Part model, mm, in its own coordinate system. Give positions to 0.01 mm unless a question says otherwise; leave off trailing zeros. Order: outer loops, then holes, each group sorted by start corner. A loop starts at its lowest first (then second) coordinate and runs counter-clockwise, first axis right, second up.
1. Slice it at C-C on z = 3.5. Give the number of separate pieces and of enclosed holes in the cut face, and give its area (3 significant figures).
2. Probe line 1 (Y direction, x = 0, z = 4.5); line 2 (X direction, y = -6.5, z = 3.5). List the from-to ranges inside material, lowest first.
3. Slice it at A-A on y = 44.45. List the corners of the cut face in (x, z), and give its area (3 significant figures).
4. Slice it at D-D on x = 0. List the corners of the cut face in (y, z).
5. Drop a flat-ended pin along its axis: pin 1 Ø5.5 at (x, y) = (-44.45, 0) entering from +Z. Give the stop position or say it passes through.
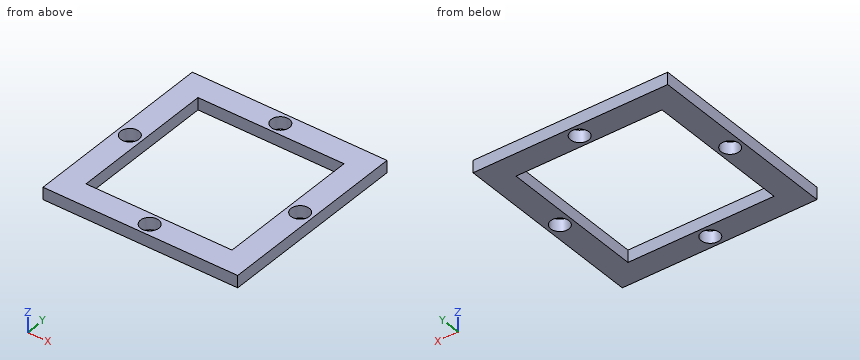
from build123d import *

# Parameters (mm, degrees)
F0_W     = 101.6
F0_H     = 101.6
F0_W_2   = 76.2
F0_H_2   = 76.2
F1_DEPTH = 6.35
F3_D     = 9.525
F3_DEPTH = 12.7


with BuildPart() as f1:
    # F0 (on Top) → F1 (new body)
    with BuildSketch(Plane.XY):
        Rectangle(F0_W, F0_H)
        Rectangle(F0_W_2, F0_H_2, mode=Mode.SUBTRACT)
    extrude(amount=F1_DEPTH)

    # F3
    with Locations(Plane.XY.offset(6.35)):
        with Locations((0, 44.45), (-44.45, 0), (44.45, 0), (0, -44.45)):
            Hole(F3_D / 2, depth=F3_DEPTH)


solid = f1.part
Data:
1. separate pieces: 1
1. enclosed holes: 5
1. area: 4,230 mm2
2. line 1: y = -50.8 to -49.21, -39.69 to -38.1, 38.1 to 39.69, 49.21 to 50.8
2. line 2: x = -50.8 to -38.1, 38.1 to 50.8
3. outline: (-50.8, 0) - (-4.76, 0) - (-4.76, 6.35) - (-50.8, 6.35) - close; (4.76, 0) - (50.8, 0) - (50.8, 6.35) - (4.76, 6.35) - close
3. area: 585 mm2
4. outline: (-50.8, 0) - (-49.21, 0) - (-49.21, 6.35) - (-50.8, 6.35) - close; (-39.69, 0) - (-38.1, 0) - (-38.1, 6.35) - (-39.69, 6.35) - close; (38.1, 0) - (39.69, 0) - (39.69, 6.35) - (38.1, 6.35) - close; (49.21, 0) - (50.8, 0) - (50.8, 6.35) - (49.21, 6.35) - close
5. pin 1: passes through
